Part print with two shaded views. Sizes in mm from the minimum x, y, z corner. Coordinates: 2 decimals unless noted, no trailing zeros. Loops run counter-clockwise (first coordinate to the right, second up) from the corner with the lowest first, then second, coordinate; pieces in that order, holes last. Notation, with made-up numbers: M -16.75,56.25 L 0.25,56.25 A27 cw 0.25,80.25 Z; hole C -39,14.5 d2. An arc over 180 degrees is marked long. Use CSV: the item, a comma, the result in double quotes. Start each with the question number.
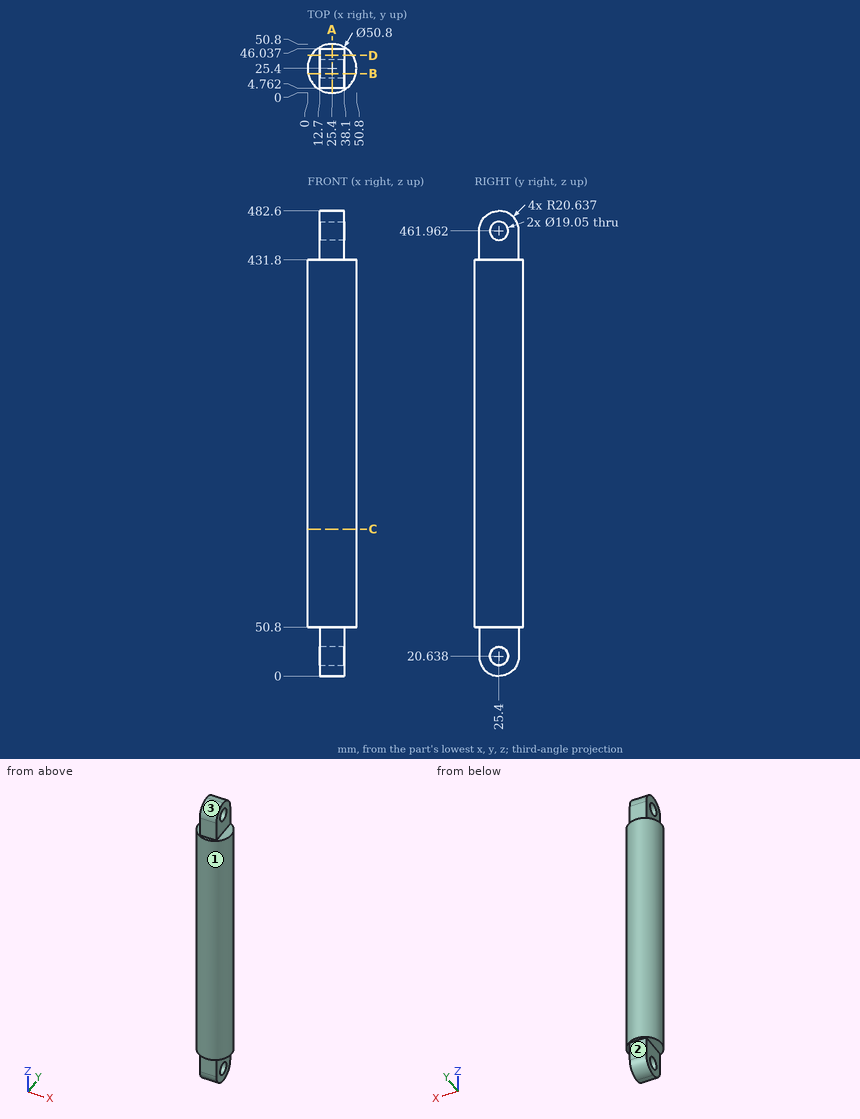
1. Pin check, flat tips, straight feed: pin 1 (1.5 mm diameter, centred on x = 16, y = 21, fed in from -Z) (1 decimal); pin 2 (5 mm diameter, centred on x = 45, y = 16, fed in from +Z); pin 3 (20.5 mm diameter, centred on y = 22.5, z = 23.5, fed in from +X). Stop position of each tip, or through.
2. Slice it at D-D, the plane y = 39. List the corners of the cut face in (x, z) (1 decimal), and give its area (3 significant figures).
3. Slice it at C-C, the plane z = 152.5. List the corners of the cut face in (x, y).
4. Slice it at A-A, the plane x = 25.4. State how many separate pieces and enclosed holes the cut face has, and give its area (3 significant figures).
5. Two-plate mould, pull along Y, no slides. Class the marked faces 1, 2 and 3: pulls with the +Y half, pulls with the -Y half, needs draft (parallel to the pull), parting line crosses it, or undercut.
6. Slice it at B-B, the plane y = 20. List the corners of the cut face in (x, z), and give its area (3 significant figures).
7. Wall check: probe 1 along Z at (x, y) = (28, 25) (1 decimal); probe 2 along Z at (x, y) = (28.5, 30) (1 decimal); probe 3 along X at (y, z) = (12, 34.5). Give the ranges that are in metal, low to high.
Found:
1,pin 1,"z = 0.3"
1,pin 2,"z = 431.8"
1,pin 3,"x = 38.1"
2,outline,"M 3.9,50.8 L 12.7,50.8 L 12.7,5.1 L 38.1,5.1 L 38.1,50.8 L 46.9,50.8 L 46.9,431.8 L 38.1,431.8 L 38.1,477.5 L 12.7,477.5 L 12.7,431.8 L 3.9,431.8 Z"
2,area,"18,700 mm^2"
3,outline,"C 25.4,25.4 d50.8"
4,separate pieces,"1"
4,enclosed holes,"2"
4,area,"22,600 mm^2"
5,face 1,"parting line crosses it"
5,face 2,"pulls with the +Y half"
5,face 3,"pulls with the -Y half"
6,outline,"M 0.58,50.8 L 12.7,50.8 L 12.7,28.48 L 38.1,28.48 L 38.1,50.8 L 50.22,50.8 L 50.22,431.8 L 38.1,431.8 L 38.1,454.12 L 12.7,454.12 L 12.7,431.8 L 0.58,431.8 Z; M 12.7,0.72 L 38.1,0.72 L 38.1,12.79 L 12.7,12.79 Z; M 12.7,469.81 L 38.1,469.81 L 38.1,481.88 L 12.7,481.88 Z"
6,area,"20,700 mm^2"
7,probe 1,"0 to 11.1, 30.2 to 452.4, 471.5 to 482.6"
7,probe 2,"0.5 to 12.3, 29 to 453.6, 470.3 to 482.1"
7,probe 3,"12.7 to 38.1"
